CAD build for the part. Positions are in the model's coordinates, mm. A direction names the side the tool comes from. Coordinates: 2 decimals unless noted, no trailing zeros. Order: outer loops, then holes, each group sorted by start corner. A loop starts at its lowest first (then second) coordinate and runs counter-clockwise, first axis right, second up. Notation, with made-up numbers: (12.5, 55.5) - (34.5, 55.5) arc R9 ccw to (34.5, 71.5) - close; hole circle Ø10 at (-10.75, -31.5). An arc over 180 degrees is marked (long way). Write each question's results on one line, items separated by ' | '. Start each with the question number.
Q1. Wall check: probe 1 along Z at (x, y) = (2.5, 7.25) (1 decimal); probe 2 along Z at (x, y) = (-15, 0.45); probe 3 along X at (y, z) = (18.75, 11). Give the ranges that are in metal, low to high.
Q2. Band-saw the part on C-C, the plane x = 2.5. Count the separate pieces of the cut face and the enclosed holes in it, then the cut area to 3 significant figures.
Q3. Pull direction Y, two halves, no side cores. Call faces 1 (the flat face through (-18, 1, -4.069)), 2 (the cylindrical face through (8.49, 25.55, 5.85)), 3 (the flat face through (9.5, 18, 8)), 4 (the flat face through (10, 30, 1)): released by +Y, released by -Y, zero draft, split by the parting line, or undercut.
Q4. Which spindle directions (+Z, -Z, +X, -X, +Y, -Y) get a long thin tool onto all of the face, cutting with end or side? Do faces 5 (the cylindrical face through (9.53, 29.4, -16.93)), 6 (the flat face through (0, 10.8, -14)), 7 (the flat face through (0, 5, 11.438)). Say none if no direction does.
Q5. Band-saw the part on B-B, the plane z = -8. Write the cut outline in (x, y).
Q6. Band-saw the part on A-A, the plane y = 18.3. Write the cut outline in (x, z), then the cut area to 3 significant figures.
Q7. Pin check, flat tips, straight feed: P1, Ø10, axis at x = -18, z = 3.5, coming from the +Y side; P2, Ø5, axis at x = -2.5, z = -13.5, coming from the +Y side; P3, Ø1, axis at y = 14.5, z = -9, coming from the -X side; P4, Ø4.5, axis at x = -25, z = 10.96, coming from the +Y side. Stop position of each tip, or through.
Autodesk Inventor part; units mm, degrees
ref_plane "YZ Plane" through (0, 0, 0) normal (1, 0, 0) x (0, 1, 0)
ref_plane "XZ Plane" through (0, 0, 0) normal (0, 1, 0) x (-1, 0, 0)
ref_plane "XY Plane" through (0, 0, 0) normal (0, 0, 1) x (1, 0, 0)
sketch "Sketch1" plane through (0, 0, 0) normal (0, 1, 0) x (-1, 0, 0)
  line L0 (6, 11.4375) -> (-6, 11.4375)
  line L1 (-6, 11.4375) -> (-6, -11.4375)
  line L2 (-6, -11.4375) -> (6, -11.4375)
  line L3 (6, -11.4375) -> (6, 11.4375)
  line L4 (6, 11.4375) -> (-6, -11.4375) construction
  line L5 (-6, 11.4375) -> (6, -11.4375) construction
  line L6 (6, 16.15) -> (-6, 16.15)
  line L7 (-6, 16.15) -> (-6, -16.15)
  line L8 (-6, -16.15) -> (6, -16.15)
  line L9 (6, -16.15) -> (6, 16.15)
  line L10 (6, 16.15) -> (-6, -16.15) construction
  line L11 (-6, 16.15) -> (6, -16.15) construction
  circle A0 centre (0, -5.4375) radius 2.5
  circle A1 centre (-2.5, 17.225) radius 2.5
  line L12 (7.5, 17.5) -> (-7.5, 17.5)
  line L13 (-7.5, 17.5) -> (-7.5, -17.5)
  line L14 (-7.5, -17.5) -> (7.5, -17.5)
  line L15 (7.5, -17.5) -> (7.5, 17.5)
  line L16 (7.5, 17.5) -> (-7.5, -17.5) construction
  line L17 (-7.5, 17.5) -> (7.5, -17.5) construction
  line L18 (7.5, 17.5) -> (-7.5, 17.5)
  line L19 (-7.5, 17.5) -> (-7.5, 29.3625)
  line L20 (-7.5, 29.3625) -> (7.5, 29.3625)
  line L21 (7.5, 29.3625) -> (7.5, 17.5)
  circle A2 centre (15, 0.9625) radius 2.5
  circle A3 centre (15, 10.9625) radius 2.5
  circle A4 centre (25, 10.9625) radius 2.5
  circle A5 centre (25, 0.9625) radius 2.5
  line L22 (28.6005, 5.9313) -> (28.6005, -4.0687)
  line L23 (28.6005, -4.0687) -> (7.5, -4.0687)
  line L24 (28.6005, 5.9313) -> (28.6005, 15.9313)
  line L25 (28.6005, 15.9313) -> (7.5, 15.9313)
  line L26 (-7.5, -17.5) -> (-11.5, -17.5)
  line L27 (-11.5, -17.5) -> (-11.5, 29.3625)
  line L28 (-11.5, 29.3625) -> (-7.5, 29.3625)
  line L29 (-7.5, 29.3625) -> (-7.5, -17.5)
  point P0 (0, 0)
  point P1 (0, -11.4375)
  point P2 (-0.2429, 16.15)
  point P3 (-4.7571, 16.15)
  point P4 (-4.9848, 17.5)
  point P5 (-0.0152, 17.5)
  dimension "d2" = 12
  dimension "d3" = 22.875
  dimension "d4" = 12
  dimension "d5" = 32.3
  dimension "d6" = 5
  dimension "d7" = 6
  dimension "d8" = 5
  dimension "d9" = 22.8
  dimension "d10" = 15
  dimension "d11" = 35
  dimension "d17" = 5
  dimension "d18" = 15
  dimension "d19" = 6.4
  dimension "d20" = 5
  dimension "d21" = 10
  dimension "d22" = 5
  dimension "d23" = 10
  dimension "d25" = 5
  dimension "d27" = 10
  dimension "d31" = 4
  dimension "d46" = 10
extrude "Extrusion1" add sketch "Sketch1" along normal blind 10.8 contours L0 L7 L6 A1 L9 | L9 L8 L7 L2
extrude "Extrusion2" add sketch "Sketch1" along normal blind 13.3 contours L9 L6 A1 L12 L15 L14 L13 L7 L1 L8 L3 | L12 L19 L20 L21 A1
extrude "Extrusion3" add sketch "Sketch1" along normal blind 2 contours L25 L24 L22 L23 L15
fillet "Fillet1" radius 2 6 edges at (-7.5, 1, -4.0687) (-7.5, 1, 15.9313) (-28.6005, 1, 15.9313) (-28.6005, 1, -4.0687) (-7.5, 6.65, 29.3625) (-7.5, 6.65, -17.5)
extrude "Extrusion4" add sketch "Sketch1" along normal blind 30 contours L13 L26 L27 L28 L19
sketch "Sketch2" plane through (7.5, 13.3, 29.3625) normal (-1, 0, 0) x (0, 0, 1)
  circle A0 centre (-23.4313, 5) radius 1.6
  circle A1 centre (-23.4313, 5) radius 2.75
  circle A2 centre (-23.4313, 15) radius 1.6
  circle A3 centre (-23.4313, 15) radius 2.75
  line L0 (0, 0) -> (-46.8625, 0)
  point P0 (-29.3625, -13.3)
  dimension "d34" = 3.2
  dimension "d35" = 5.5
  dimension "d36" = 3.2
  dimension "d37" = 5.5
  dimension "d39" = 5
  dimension "d40" = 10
extrude "Extrusion5" cut sketch "Sketch2" against normal blind 4 contours A0 | A2
extrude "Extrusion6" cut sketch "Sketch2" against normal blind 2
fillet "Fillet2" radius 2 2 edges at (9.5, 30, 29.3625) (9.5, 30, -17.5)
properties part number "Bracket Servo_3DPrint"
Results below:
1) probe 1: z = -17.5 to -11.4, 11.4 to 14.7, 19.7 to 29.4 | probe 2: z = -4.07 to -1.54, 3.46 to 8.46, 13.46 to 15.93 | probe 3: x = 7.5 to 11.5
2) separate pieces: 3 | enclosed holes: 0 | area: 233 mm²
3) face 1: zero draft | face 2: undercut | face 3: undercut | face 4: released by +Y
4) face 5: -Z, +X, -X, +Y | face 6: +Y | face 7: +Y, -Y
5) outline: (-7.5, 0) - (-6, 0) - (-6, 13.3) - (-7.5, 13.3) - close; (6, 0) - (11.5, 0) - (11.5, 30) - (7.5, 30) - (7.5, 13.3) - (6, 13.3) - close
6) outline: (7.5, -17.5) - (11.5, -17.5) - (11.5, 4.33) - (9.5, 4.33) - (9.5, 3.18) - (7.5, 3.18) - close; (7.5, 8.68) - (9.5, 8.68) - (9.5, 7.53) - (11.5, 7.53) - (11.5, 29.36) - (7.5, 29.36) - close | area: 170 mm²
7) P1: stops at y = 2 | P2: stops at y = 10.8 | P3: stops at x = 7.5 | P4: passes through
